Geometry check sheet. Reference: the model listing, model coordinates, mm. Face numbers are marked on the shaded views. Coordinates: 2 decimals unless noted, no trailing zeros. Write each loop counter-clockwise with the first axis right and the second up, starting at its lowest first coordinate (ties: lowest second). Pieces come first, ordered by that corner, then holes. Notation, with made-up numbers: (57, 84) -> (106, 84) arc R30 cw to (106, 111) -> close; hole circle Ø2 at (-11, -29.75). An arc over 180 degrees is marked (long way). Answer in a Markdown table with one row per item. Add a question column.
1. Mould release check, pull along Y, two halves, no side actions. Record for the marked faces 1, 2 and 3: pulls with the +Y half, pulls with the -Y half, needs draft (parallel to the pull), parting line crosses it, or undercut.
2. Cross-section at B-B on y = 1.75. Record the cut outline in (x, z), and give its area (3 significant figures).
3. Cross-section at A-A on x = 7.5. Record the cut outline in (y, z), and give its area (3 significant figures).
4. Cross-section at C-C on x = 10.5. Record the cut outline in (y, z), and give its area (3 significant figures).
5. Scan lines: L1, parallel to Y at x = 7.5, z = -0.8; L2, parallel to Z at x = 2.75, y = 3.5; L3, parallel to Y at x = 7.5, z = 0.1. Record each from-to range of solid material in increasing order. Write a range as from..to.
6. Cross-section at D-D on z = 0.2. Record the cut outline in (x, y), and give its area (3 significant figures).
```python
from build123d import *

# Parameters (mm, degrees)
SKETCH1_W           = 15
SKETCH1_H           = 9.998
BOSS_EXTRUDE1_DEPTH = 1.65
SKETCH2_R           = 2.6
BOSS_EXTRUDE2_DEPTH = 1.65
SKETCH3_R           = 2.4
CUT_EXTRUDE1_DEPTH  = 4.3
FILLET1_R           = 0.1
FILLET3_R           = 0.5
FILLET4_R           = 0.5


with BuildPart() as part:
    # Sketch1 → Boss-Extrude1 (new body)
    with BuildSketch(Plane.XY):
        with Locations((7.5, 4.999)):
            Rectangle(SKETCH1_W, SKETCH1_H)
    extrude(amount=BOSS_EXTRUDE1_DEPTH)

    # Sketch2 → Boss-Extrude2 (add)
    with BuildSketch(Plane(origin=(0, 0, 0), x_dir=(-1, 0, 0), z_dir=(0, 0, -1))):
        with Locations((-7.5, 4.999)):
            Circle(SKETCH2_R)
    extrude(amount=BOSS_EXTRUDE2_DEPTH)

    # Sketch3 → Cut-Extrude1 (cut, through all)
    with BuildSketch(Plane.XY.offset(1.65)):
        with Locations((7.5, 4.999)):
            Circle(SKETCH3_R)
    extrude(amount=-CUT_EXTRUDE1_DEPTH, mode=Mode.SUBTRACT)

    # Fillet1
    fillet1_edges = [part.edges().sort_by_distance(p)[0] for p in [
        (10.1, 4.999, 0),
        (10.1, 4.999, -1.65),
        (5.1, 4.999, 1.65),
    ]]
    fillet(fillet1_edges, radius=FILLET1_R)

    # Fillet3
    fillet3_edges = [part.edges().sort_by_distance(p)[0] for p in [
        (0, 0, 0.825),
        (0, 9.998, 0.825),
        (15, 9.998, 0.825),
        (15, 0, 0.825),
    ]]
    fillet(fillet3_edges, radius=FILLET3_R)

    # Fillet4
    fillet4_edges = [part.edges().sort_by_distance(p)[0] for p in [
        (7.5, 9.998, 0),
        (7.5, 9.998, 1.65),
        (7.5, 0, 0),
        (0, 4.999, 0),
        (15, 4.999, 0),
        (0.146446609, 0.146446609, 0),
        (0.146446609, 9.851553391, 0),
        (14.853553391, 0.146446609, 0),
        (14.853553391, 9.851553391, 0),
        (15, 4.999, 1.65),
        (7.5, 0, 1.65),
        (0, 4.999, 1.65),
        (0.146446609, 0.146446609, 1.65),
        (0.146446609, 9.851553391, 1.65),
        (14.853553391, 0.146446609, 1.65),
        (14.853553391, 9.851553391, 1.65),
    ]]
    fillet(fillet4_edges, radius=FILLET4_R)


solid = part.part
```
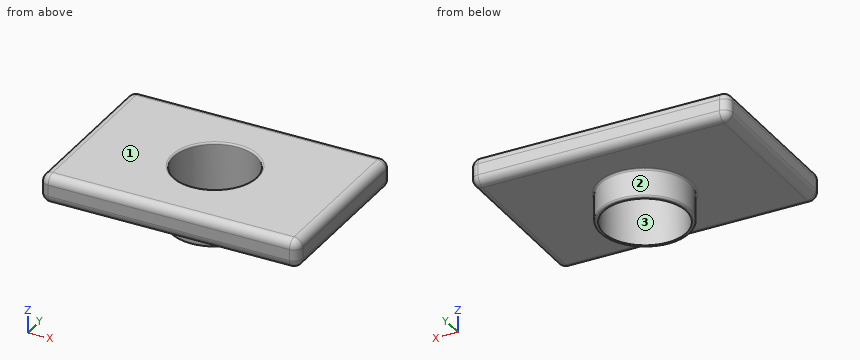
Results found:
| question | item | result |
|---|---|---|
| 1 | face 1 | needs draft |
| 1 | face 2 | parting line crosses it |
| 1 | face 3 | undercut |
| 2 | outline | (0, 0.5) arc R0.5 ccw to (0.5, 0) -> (14.5, 0) arc R0.5 ccw to (15, 0.5) -> (15, 1.15) arc R0.5 ccw to (14.5, 1.65) -> (0.5, 1.65) arc R0.5 ccw to (0, 1.15) -> close |
| 2 | area | 24.5 mm^2 |
| 3 | outline | (0, 0.5) arc R0.5 ccw to (0.5, 0) -> (2.3, 0) arc R0.1 cw to (2.4, -0.1) -> (2.4, -1.55) arc R0.1 ccw to (2.5, -1.65) -> (2.6, -1.65) -> (2.6, 1.55) arc R0.1 ccw to (2.5, 1.65) -> (0.5, 1.65) arc R0.5 ccw to (0, 1.15) -> close; (7.4, -1.65) -> (7.5, -1.65) arc R0.1 ccw to (7.6, -1.55) -> (7.6, -0.1) arc R0.1 cw to (7.7, 0) -> (9.5, 0) arc R0.5 ccw to (10, 0.5) -> (10, 1.15) arc R0.5 ccw to (9.5, 1.65) -> (7.5, 1.65) arc R0.1 ccw to (7.4, 1.55) -> close |
| 3 | area | 9.02 mm^2 |
| 4 | outline | (0, 0.5) arc R0.5 ccw to (0.5, 0) -> (9.5, 0) arc R0.5 ccw to (10, 0.5) -> (10, 1.15) arc R0.5 ccw to (9.5, 1.65) -> (0.5, 1.65) arc R0.5 ccw to (0, 1.15) -> close |
| 4 | area | 16.3 mm^2 |
| 5 | L1 | y = 2.4..2.6, 7.4..7.6 |
| 5 | L2 | z = 0..1.65 |
| 5 | L3 | y = 0.2..2.6, 7.4..9.8 |
| 6 | outline | (0.1, 0.5) arc R0.4 ccw to (0.5, 0.1) -> (14.5, 0.1) arc R0.4 ccw to (14.9, 0.5) -> (14.9, 9.5) arc R0.4 ccw to (14.5, 9.9) -> (0.5, 9.9) arc R0.4 ccw to (0.1, 9.5) -> close; hole circle Ø4.8 at (7.5, 5) |
| 6 | area | 127 mm^2 |
